The listing builds one solid part. Answer for the finished solid, in the listing's coordinates (mm). Face numbers are marked on the shaded views. A direction names the side the tool comes from. Coordinates: 2 decimals unless noted, no trailing zeros. Loops run counter-clockwise (first coordinate to the right, second up) from the corner with the lowest first, then second, coordinate; pieces in that order, holes last. Notation, with made-up numbers: (-27, 79) -> (18, 79) arc R17 ccw to (18, 88) -> close; hole circle Ø2 at (39.5, 0). An arc over 180 degrees is marked (long way). Answer in a Markdown table with one row per item.
```python
from build123d import *

# Parameters (mm, degrees)
F0_W     = 50
F0_H     = 25
F1_DEPTH = 25
F2_R     = 5
F3_T     = -2.5


# Not quite as in the source:
# - a shell that OpenCascade refuses in one call is made with other operations: the cavity is built on its own and cut out


with BuildPart() as f1:
    # F0 (on Top) → F1 (new body)
    with BuildSketch(Plane.XY):
        with Locations((-25, 12.5)):
            Rectangle(F0_W, F0_H)
    extrude(amount=F1_DEPTH)

    # F2
    f2_edges = [f1.edges().sort_by_distance(p)[0] for p in [
        (0, 12.5, 25),
        (-25, 0, 25),
        (-50, 12.5, 25),
        (-25, 25, 25),
        (-50, 25, 12.5),
        (-50, 12.5, 0),
        (-50, 0, 12.5),
        (-25, 0, 0),
        (0, 12.5, 0),
        (-25, 25, 0),
        (0, 25, 12.5),
        (0, 0, 12.5),
    ]]
    fillet(f2_edges, radius=F2_R)

    # F3: a shell. OpenCascade refuses it in one call, so the cavity is built on its own and cut out:
    # the body offset inwards by the wall thickness, plus a prism from it out through each open face.
    f3_core = offset(f1.part, amount=F3_T, mode=Mode.PRIVATE)
    f3_exits = [f3_core.faces().sort_by_distance(p)[0] for p in [
        (-25, 12.5, 22.5),
    ]]
    add(f3_core, mode=Mode.SUBTRACT)
    extrude(f3_exits, amount=-F3_T, mode=Mode.SUBTRACT)


solid = f1.part
```
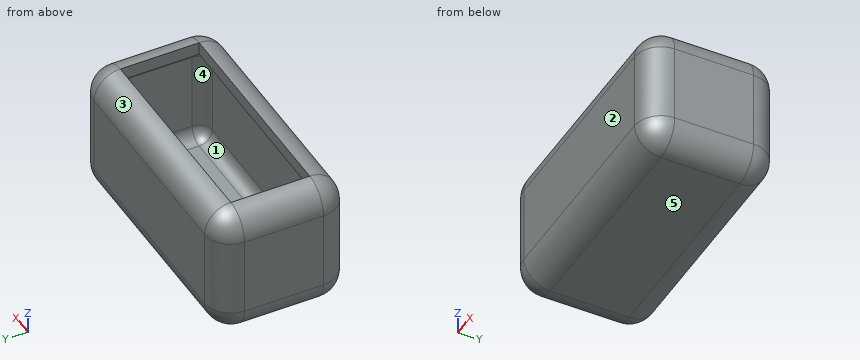
Item 1: Find the intervals of material crossed by probe 1 along Y at (x, z) = (-31, 17.5); probe 2 along X at (y, z) = (16, 5.5); probe 3 along Z at (x, y) = (-42.5, 15.25), in increasing order.
Findings below:
| item | result |
|---|---|
| probe 1 | y = 0 to 2.5, 22.5 to 25 |
| probe 2 | x = -50 to -47.5, -2.5 to 0 |
| probe 3 | z = 0 to 2.5 |
Item 2: A cutting plane is placed at B-B, the plane y = 20.75. Determine the outline of the cut face in (x, z), plus the area to 3 significant figures.
Findings below:
| item | result |
|---|---|
| outline | (-49.94, 5) arc R4.94 ccw to (-45, 0.06) -> (-5, 0.06) arc R4.94 ccw to (-0.06, 5) -> (-0.06, 20) arc R4.94 ccw to (-5, 24.94) -> (-45, 24.94) arc R4.94 ccw to (-49.94, 20) -> close; hole (-47.38, 5) arc R2.38 ccw to (-45, 2.62) -> (-5, 2.62) arc R2.38 ccw to (-2.62, 5) -> (-2.62, 20) arc R2.38 ccw to (-5, 22.38) -> (-45, 22.38) arc R2.38 ccw to (-47.38, 20) -> close |
| area | 340 mm2 |
Item 3: A cutting plane is placed at A-A, the plane z = 23. Determine the outline of the cut face in (x, y).
Findings below:
| item | result |
|---|---|
| outline | (-49, 5) arc R4 ccw to (-45, 1) -> (-5, 1) arc R4 ccw to (-1, 5) -> (-1, 20) arc R4 ccw to (-5, 24) -> (-45, 24) arc R4 ccw to (-49, 20) -> close; hole (-45, 5) -> (-5, 5) -> (-5, 20) -> (-45, 20) -> close |
Item 4: Determine the mould class of the marked faces 1, 2 and 3 for opening direction Y: +Y half, -Y half, draft (parallel to the pull), parting line (faces both ways), or undercut.
Findings below:
| item | result |
|---|---|
| face 1 | undercut |
| face 2 | -Y half |
| face 3 | +Y half |
Item 5: A tool of negligible diameter and unlimited length cuts with its end or side. For the marked faces 4 and 5, from which of +Z, -Z, +X, -X, +Y, -Y can it reach the whole face along a straight path? Write none if from no direction.
Findings below:
| item | result |
|---|---|
| face 4 | none |
| face 5 | -Z, +X, -X, +Y, -Y |
Item 6: Flat-ended cylindrical pins translate along their axes: pin 1 Ø2 at (y, z) = (11.5, 24) entering from +X; pin 2 Ø1.2 at (x, z) = (-24.5, 24) entering from +Y; pin 3 Ø4 at (y, z) = (15, 4) entering from +X; pin 4 Ø3 at (x, z) = (-16, 24) entering from -Y. Find the tip coordinate at first contact, or state that the pin passes through.
Findings below:
| item | result |
|---|---|
| pin 1 | stops at x = -1 |
| pin 2 | stops at y = 23.67 |
| pin 3 | stops at x = 0 |
| pin 4 | stops at y = 0.67 |
Item 7: A cutting plane is placed at C-C, the plane x = -13. Determine the outline of the cut face in (y, z), plus the area to 3 significant figures.
Findings below:
| item | result |
|---|---|
| outline | (0, 5) arc R5 ccw to (5, 0) -> (20, 0) arc R5 ccw to (25, 5) -> (25, 20) arc R5 ccw to (20, 25) -> (20, 22.5) arc R2.5 cw to (22.5, 20) -> (22.5, 5) arc R2.5 cw to (20, 2.5) -> (5, 2.5) arc R2.5 cw to (2.5, 5) -> (2.5, 20) arc R2.5 cw to (5, 22.5) -> (5, 25) arc R5 ccw to (0, 20) -> close |
| area | 171 mm2 |
Item 8: A cutting plane is placed at D-D, the plane z = 19.5. Determine the outline of the cut face in (x, y), plus the area to 3 significant figures.
Findings below:
| item | result |
|---|---|
| outline | (-50, 5) arc R5 ccw to (-45, 0) -> (-5, 0) arc R5 ccw to (0, 5) -> (0, 20) arc R5 ccw to (-5, 25) -> (-45, 25) arc R5 ccw to (-50, 20) -> close; hole (-47.5, 5) arc R2.5 ccw to (-45, 2.5) -> (-5, 2.5) arc R2.5 ccw to (-2.5, 5) -> (-2.5, 20) arc R2.5 ccw to (-5, 22.5) -> (-45, 22.5) arc R2.5 ccw to (-47.5, 20) -> close |
| area | 334 mm2 |
